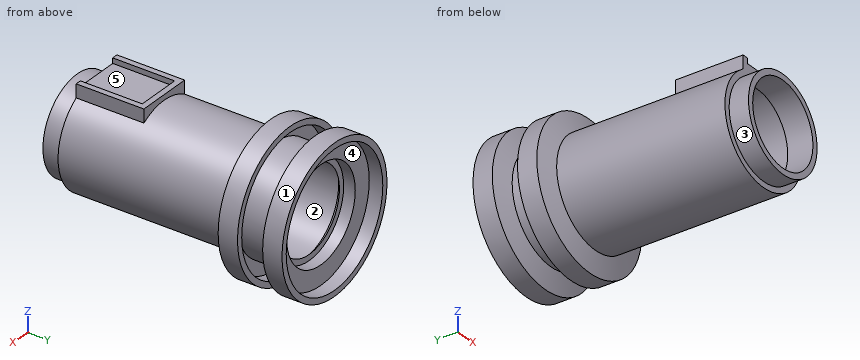
```python
from build123d import *

# Parameters (mm, degrees)
SALIENTE_EXTRUIR1_DEPTH = 35
CROQUIS3_W              = 23.109686168
CROQUIS3_H              = 32
CORTAR_EXTRUIR1_DEPTH   = 2.7


with BuildPart() as part:
    # Croquis1 → Revolución1 (revolve)
    with BuildSketch(Plane.XY):
        Polygon((-39.212995514, 3.519897437), (-39.212995514, 16.519897437), (-42.212995514, 16.519897437), (-42.212995514, 120.917625562), (-39.212995514, 123.519897437), (-42.212995514, 123.519897437), (-42.212995514, 129.519897437), (-52.212995514, 129.519897437), (-52.212995514, 136.519897437), (-55.212995514, 136.519897437), (-55.212995514, 126.519897437), (-45.212995514, 123.519897437), (-45.212995514, 106.519897437), (-52.212995514, 106.519897437), (-52.212995514, 113.519897437), (-55.212995514, 113.519897437), (-55.212995514, 103.519897437), (-45.212995514, 100.519897437), (-45.212995514, 13.519897437), (-42.212995514, 13.519897437), (-42.212995514, 3.519897437), align=None)
    revolve(axis=Axis((-17.712995514, 104.262295082, 0), (0, -1, 0)))

    # Croquis2 → Saliente-Extruir1 (add)
    with BuildSketch(Plane.XZ.offset(-13.519897437)):
        with BuildLine():
            Line((-32.267838598, 23.332521141), (-32.267838598, 30.202521141))
            Line((-32.267838598, 30.202521141), (-3.15815243, 30.202521141))
            Line((-3.15815243, 30.202521141), (-3.15815243, 23.332521141))
            ThreePointArc((-3.15815243, 23.332521141), (-17.712995514, 27.5), (-32.267838598, 23.332521141))
        make_face()
    extrude(amount=-SALIENTE_EXTRUIR1_DEPTH)

    # Croquis3 → Cortar-Extruir1 (cut)
    with BuildSketch(Plane.XY.offset(30.202521141)):
        with Locations((-17.712995514, 29.519897437)):
            Rectangle(CROQUIS3_W, CROQUIS3_H)
    extrude(amount=-CORTAR_EXTRUIR1_DEPTH, mode=Mode.SUBTRACT)


solid = part.part
```
Part model, mm, in its own coordinate system. Face numbers are marked on the shaded views. A direction names the side the tool comes from. Give positions to 0.01 mm unless a question says otherwise; leave off trailing zeros. Use one line per item in the form item = value.
Item 1: Two-plate mould, pull along Z, no slides. Class the marked faces 3, 4 and 5: released by +Z, released by -Z, zero draft, split by the parting line, or undercut.
Solution:
face_3 = split by the parting line
face_4 = undercut
face_5 = released by +Z
Item 2: Pin check, flat tips, straight feed: pin 1 Ø12 at (x, y) = (1, 18.5) entering from -Z; pin 2 Ø2 at (y, z) = (25, 26.5) entering from -X; pin 3 Ø1 at (x, z) = (-46, 15.5) entering from +Y. Stop position of each tip, or through.
Solution:
pin_1 = -24.39
pin_2 = -32.27
pin_3 = 129.52
Item 3: Probe probe 1 along X at (y, z) = (45, 0); probe 2 along X at (y, z) = (132, 0); probe 3 along X at (y, z) = (113, -4.5). List the from-to ranges inside material, lowest first. Write a range as from..to.
Solution:
probe_1 = -45.21..-42.21, 6.79..9.79
probe_2 = -55.21..-52.21, 16.79..19.79
probe_3 = -54.94..-51.92, -44.84..-41.8, 6.37..9.42, 16.49..19.52
Item 4: Which spindle directions (+Z, -Z, +X, -X, +Y, -Y) get a long thin tool onto all of the face, cutting with end or side? Do the marked faces 1 and 2. Say none if no direction does.
Solution:
face_1 = +Y, -Y
face_2 = none
